Build history of the part. All positions in model axes, mm. Face numbers are marked on the shaded views. A direction names the side the tool comes from. Give positions to 0.01 mm unless a question says otherwise; leave off trailing zeros. Order: outer loops, then holes, each group sorted by start corner. A loop starts at its lowest first (then second) coordinate and runs counter-clockwise, first axis right, second up. Notation, with made-up numbers: (76, 7) - (133, 7) arc R21 cw to (133, 27) - close; hole circle Ø3 at (59.5, 74.5). An arc over 180 degrees is marked (long way). Answer in a Markdown table with one row per item.
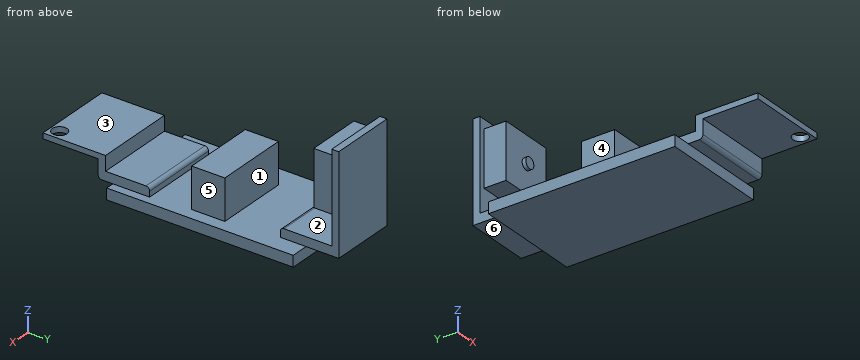
```python
from build123d import *

# Parameters (mm, degrees)
SKETCH_W      = 29.3
SKETCH_H      = 50.7
PAD_DEPTH     = 3
SKETCH001_W   = 18
SKETCH001_H   = 14
SKETCH001_W_2 = 22
PAD001_DEPTH  = 2.5
FILLET_R      = 1
SKETCH002_W   = 18
SKETCH002_H   = 27
PAD002_DEPTH  = 1.9
SKETCH003_W   = 15
SKETCH003_H   = 15
PAD003_DEPTH  = 6
SKETCH004_R   = 1.5
PAD004_DEPTH  = 1
SKETCH005_W   = 22
SKETCH005_H   = 2
PAD005_DEPTH  = 2.5
SKETCH006_W   = 22
SKETCH006_H   = 17
PAD006_DEPTH  = 1.5
SKETCH007_R   = 2
POCKET_DEPTH  = 5
SKETCH008_W   = 20
SKETCH008_H   = 9
PAD007_DEPTH  = 11
FILLET001_R   = 1


with BuildPart() as part:
    # Sketch → Pad (new body)
    with BuildSketch(Plane.XY):
        Rectangle(SKETCH_W, SKETCH_H)
    extrude(amount=PAD_DEPTH)

    # Sketch001 → Pad001 (new body)
    with BuildSketch(Plane.XY.offset(3)):
        with Locations((0.85, 25.35)):
            Rectangle(SKETCH001_W, SKETCH001_H)
        with Locations((1.35, -22.35)):
            Rectangle(SKETCH001_W_2, SKETCH001_H)
    extrude(amount=PAD001_DEPTH)

    # Fillet
    fillet_edges = [part.edges().sort_by_distance(p)[0] for p in [
        (0.85, 18.35, 5.5),
        (1.35, -15.35, 5.5),
    ]]
    fillet(fillet_edges, radius=FILLET_R)

    # Sketch002 → Pad002 (new body)
    with BuildSketch(Plane(origin=(0, 32.35, 0), x_dir=(-1, 0, 0), z_dir=(0, 1, 0))):
        with Locations((-0.85, 16.5)):
            Rectangle(SKETCH002_W, SKETCH002_H)
    extrude(amount=PAD002_DEPTH)

    # Sketch003 → Pad003 (new body)
    with BuildSketch(Plane.XZ.offset(-32.35)):
        with Locations((0.85, 20)):
            Rectangle(SKETCH003_W, SKETCH003_H)
    extrude(amount=PAD003_DEPTH)

    # Sketch004 → Pad004 (new body)
    with BuildSketch(Plane.XZ.offset(-26.35)):
        with Locations((0.85, 20)):
            Circle(SKETCH004_R)
    extrude(amount=PAD004_DEPTH)

    # Sketch005 → Pad005 (new body)
    with BuildSketch(Plane.XY.offset(5.5)):
        with Locations((1.35, -28.35)):
            Rectangle(SKETCH005_W, SKETCH005_H)
    extrude(amount=PAD005_DEPTH)

    # Sketch006 → Pad006 (new body)
    with BuildSketch(Plane.XY.offset(8)):
        with Locations((1.35, -35.85)):
            Rectangle(SKETCH006_W, SKETCH006_H)
    extrude(amount=PAD006_DEPTH)

    # Sketch007 → Pocket (cut)
    with BuildSketch(Plane.XY.offset(9.5)):
        with Locations((9.55, -41.85)):
            Circle(SKETCH007_R)
    extrude(amount=-POCKET_DEPTH, mode=Mode.SUBTRACT)

    # Sketch008 → Pad007 (new body)
    with BuildSketch(Plane.XY.offset(3)):
        with Locations((1.35, -0.15)):
            Rectangle(SKETCH008_W, SKETCH008_H)
    extrude(amount=PAD007_DEPTH)

    # Fillet001
    fillet001_edges = [part.edges().sort_by_distance(p)[0] for p in [
        (1.35, -29.35, 3),
    ]]
    fillet(fillet001_edges, radius=FILLET001_R)


solid = part.part
```
1. Probe line 1 (Y direction, x = 9.55, z = 8.6); line 2 (Y direction, x = -1, z = 4.25); line 3 (Y direction, x = -8.5, z = 6). List the from-to ranges inside material, lowest first.
Check result:
| item | result |
|---|---|
| line 1 | y = -44.35 to -43.85, -39.85 to -27.35, -4.65 to 4.35, 32.35 to 34.25 |
| line 2 | y = -29.35 to -15.35, -4.65 to 4.35, 18.35 to 34.25 |
| line 3 | y = -29.35 to -27.35, -4.65 to 4.35 |
2. Drop flat-ended pins along their axis: P1, Ø3.5, axis at x = -3.5, z = 1, coming from the +Y side; P2, Ø6, axis at x = 4.5, z = 4, coming from the -Y side; P3, Ø1, axis at x = 9, y = 25, coming from the +Z side; P4, Ø14.5, axis at x = 3, y = 28.5, coming from the +Z side. Give the stop position or say it passes through.
Check result:
| item | result |
|---|---|
| P1 | stops at y = 25.35 |
| P2 | stops at y = -29.35 |
| P3 | stops at z = 5.5 |
| P4 | stops at z = 30 |
3. Which spindle directions (+Z, -Z, +X, -X, +Y, -Y) get a long thin tool onto all of the face, cutting with end or side? Do the marked faces 4, 5 and 6. Say none if no direction does.
Check result:
| item | result |
|---|---|
| face 4 | +Z, -X, +Y |
| face 5 | +Z, +X, +Y |
| face 6 | -Z, +X, -X, +Y |
4. Cut at A-A on z = 13.25. Write the cut outline in (x, y), and give its area (3 significant figures).
Check result:
| item | result |
|---|---|
| outline | (-8.65, -4.65) - (11.35, -4.65) - (11.35, 4.35) - (-8.65, 4.35) - close; (-8.15, 32.35) - (-6.65, 32.35) - (-6.65, 26.35) - (8.35, 26.35) - (8.35, 32.35) - (9.85, 32.35) - (9.85, 34.25) - (-8.15, 34.25) - close |
| area | 304 mm² |
5. Cut at C-C on z = 16.75. Write the cut outline in (x, y).
Check result:
| item | result |
|---|---|
| outline | (-8.15, 32.35) - (-6.65, 32.35) - (-6.65, 26.35) - (8.35, 26.35) - (8.35, 32.35) - (9.85, 32.35) - (9.85, 34.25) - (-8.15, 34.25) - close |
6. Cut at B-B on y = -41.85. Write the cut outline in (x, z).
Check result:
| item | result |
|---|---|
| outline | (-9.65, 8) - (7.55, 8) - (7.55, 9.5) - (-9.65, 9.5) - close; (11.55, 8) - (12.35, 8) - (12.35, 9.5) - (11.55, 9.5) - close |
7. Two-plate mould, pull along Z, no slides. Class the marked faces 1, 2 and 3: +Z half, -Z half, draft (parallel to the pull), parting line (faces both ways), or undercut.
Check result:
| item | result |
|---|---|
| face 1 | draft |
| face 2 | undercut |
| face 3 | +Z half |
